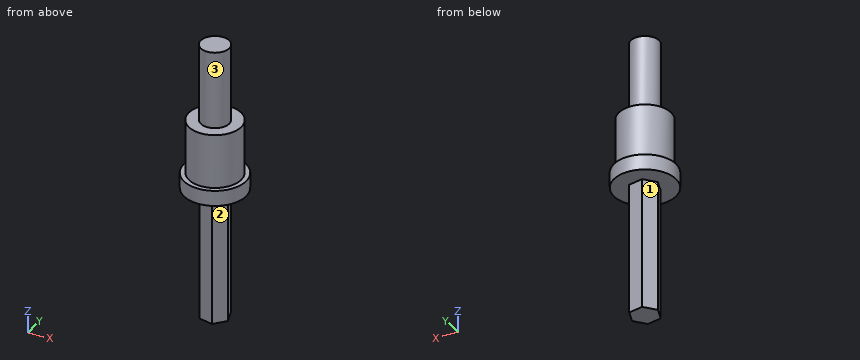
Autodesk Inventor part; units mm, degrees
ref_plane "YZ Plane" through (0, 0, 0) normal (1, 0, 0) x (0, 1, 0)
ref_plane "XZ Plane" through (0, 0, 0) normal (0, 1, 0) x (-1, 0, 0)
ref_plane "XY Plane" through (0, 0, 0) normal (0, 0, 1) x (1, 0, 0)
sketch "Sketch1" plane through (0, 0, 0) normal (0, 0, 1) x (1, 0, 0)
  circle A0 centre (0, 0) radius 4.5 construction
  line L0 (-1.8766, -2.1935) -> (-2.838, 0.5284) construction
  line L1 (-2.838, 0.5284) -> (-0.9614, 2.722) construction
  line L2 (-0.9614, 2.722) -> (1.8766, 2.1935) construction
  line L3 (1.8766, 2.1935) -> (2.838, -0.5284) construction
  line L4 (2.838, -0.5284) -> (0.9614, -2.722) construction
  line L5 (0.9614, -2.722) -> (-1.8766, -2.1935) construction
  line L6 (-0.9498, 2.6893) -> (-2.8039, 0.5221)
  line L7 (-2.8039, 0.5221) -> (-1.8541, -2.1672)
  line L8 (-1.8541, -2.1672) -> (0.9498, -2.6893)
  line L9 (0.9498, -2.6893) -> (2.8039, -0.5221)
  line L10 (2.8039, -0.5221) -> (1.8541, 2.1672)
  line L11 (1.8541, 2.1672) -> (-0.9498, 2.6893)
  dimension "d0" = 0.03
extrude "Extrusion1" add sketch "Sketch1" against normal blind 25.4
sketch "Sketch2" plane through (0, 0, 0) normal (0, 0, 1) x (1, 0, 0)
  circle A0 centre (0, 0) radius 6
  dimension "d3" = 12
extrude "Extrusion2" add sketch "Sketch2" along normal blind 3
sketch "Sketch4" plane through (0, 0, 3) normal (0, 0, 1) x (1, 0, 0)
  circle A0 centre (0, 0) radius 5.08 construction
  circle A1 centre (0, 8) radius 1.48 construction
  circle A2 centre (6.9282, 4) radius 1.48 construction
  circle A3 centre (6.9282, -4) radius 1.48 construction
  circle A4 centre (0, -8) radius 1.48 construction
  circle A5 centre (-6.9282, -4) radius 1.48 construction
  circle A6 centre (-6.9282, 4) radius 1.48 construction
  circle A7 centre (0, 0) radius 5.05
  circle A8 centre (0, 0) radius 12.7
  point P0 (0, 0)
  dimension "d7" = 0.03
extrude "Extrusion3" add sketch "Sketch4" along normal blind 10.5 contours A7
sketch "Sketch5" plane through (0, 0, 13.5) normal (0, 0, 1) x (1, 0, 0)
  circle A0 centre (0, 0) radius 2.75
  point P0 (0, 0)
  dimension "d10" = 5.5
extrude "Extrusion4" add sketch "Sketch5" along normal blind 15
properties part number "Shaft"
Geometry check sheet. Reference: the model listing, model coordinates, mm. Face numbers are marked on the shaded views. A direction names the side the tool comes from. Coordinates: 2 decimals unless noted, no trailing zeros. Order: outer loops, then holes, each group sorted by start corner. A loop starts at its lowest first (then second) coordinate and runs counter-clockwise, first axis right, second up. Notation, with made-up numbers: (1.5, 22.25) - (40.5, 22.25) arc R24 ccw to (40.5, 52.25) - close; hole circle Ø10 at (-28.5, 42.5). An arc over 180 degrees is marked (long way). Answer in a Markdown table with one row per item. Add a question column.
1. Section check D-D (x = 0). Enter the section's corners in (y, z), plus the area to 3 significant figures.
2. Gauge pin test, flat ends, axial feed: pin 1 Ø1.5 at (y, z) = (-0.5, 15.5) entering from -X; pin 2 Ø1.5 at (y, z) = (-2.5, -5.5) entering from -X; pin 3 Ø3 at (x, y) = (-1, 4.5) entering from +Z. Record the tip position at first contact, or that the pin passes through.
3. Section check A-A (x = 3.5). Enter the section's corners in (y, z).
4. Access from +Z, -Z, +X, -X, +Y, -Y to the whole of each face (thin tool, end or side, straight path). Record for the marked faces 1, 2 and 3.
5. Material ranges on L1, parallel to Z at x = 2.5, y = -3; L2, parallel to Z at x = 4.5, y = -2.5; L3, parallel to X at y = 1, z = 26, recorded low to high. Write a range as [from, to].
6. Section check C-C (z = -16). Enter the section's corners in (x, y).
Data:
| question | item | result |
|---|---|---|
| 1 | outline | (-6, 0) - (-2.51, 0) - (-2.51, -25.4) - (2.51, -25.4) - (2.51, 0) - (6, 0) - (6, 3) - (5.05, 3) - (5.05, 13.5) - (2.75, 13.5) - (2.75, 28.5) - (-2.75, 28.5) - (-2.75, 13.5) - (-5.05, 13.5) - (-5.05, 3) - (-6, 3) - close |
| 1 | area | 352 mm² |
| 2 | pin 1 | stops at x = -2.75 |
| 2 | pin 2 | stops at x = -2 |
| 2 | pin 3 | stops at z = 13.5 |
| 3 | outline | (-4.87, 0) - (4.87, 0) - (4.87, 3) - (3.64, 3) - (3.64, 13.5) - (-3.64, 13.5) - (-3.64, 3) - (-4.87, 3) - close |
| 4 | face 1 | -Z, -X, +Y |
| 4 | face 2 | -Z, +X, -Y |
| 4 | face 3 | +Z |
| 5 | L1 | z = [0, 13.5] |
| 5 | L2 | z = [0, 3] |
| 5 | L3 | x = [-2.56, 2.56] |
| 6 | outline | (-2.8, 0.52) - (-1.85, -2.17) - (0.95, -2.69) - (2.8, -0.52) - (1.85, 2.17) - (-0.95, 2.69) - close |
